Geometry: final body of the model. Coordinates: model frame, mm. A direction names the side the tool comes from. Give positions to 0.01 mm unless a question says otherwise; leave off trailing zeros. Write each loop counter-clockwise with the first axis right and the second up, starting at its lowest first coordinate (ties: lowest second). Pieces come first, ordered by that corner, then holes. Notation, with made-up numbers: (67.25, -11) -> (79.25, -11) arc R12 cw to (79.25, -3) -> close; hole circle Ø11 at (77, -12.5). An arc over 180 degrees is marked (long way). Answer as a JSON object with one key per item and string values.
from build123d import *

# Parameters (mm, degrees)
SKETCH_1_W           = 300
SKETCH_1_H           = 30
EXTRUDE_1_DEPTH      = 20
EXTRUDE_2_DEPTH      = 28
EXTRUDE_2_DEPTH_BACK = 328
SKETCH_3_R           = 4
CUT_EXTRUDE_1_DEPTH  = 182.614977356
SKETCH_3_3_R         = 6
SKETCH_3_3_R_2       = 4
CUT_EXTRUDE_2_DEPTH  = 182.614977356
SKETCH_3_4_R         = 13.5
SKETCH_3_4_R_2       = 13.25
SKETCH_3_4_R_3       = 6
CUT_EXTRUDE_3_DEPTH  = 182.614977356
SKETCH_3_5_R         = 2.4
CUT_EXTRUDE_4_DEPTH  = 4.5
SKETCH_3_6_R         = 2.4
CUT_EXTRUDE_5_DEPTH  = 5


with BuildPart() as part:
    # Sketch 1 → Extrude 1 (new body)
    with BuildSketch(Plane.XY):
        with Locations((0, 15)):
            Rectangle(SKETCH_1_W, SKETCH_1_H)
    extrude(amount=EXTRUDE_1_DEPTH)

    # Sketch 2 → Extrude 2 (add, two sides: drawn at the far end of the back side and taken through both)
    with BuildSketch(Plane.ZY.offset(150).offset(-EXTRUDE_2_DEPTH_BACK)):
        with BuildLine():
            Line((0, 20), (0, 10))
            ThreePointArc((0, 10), (5, 15), (0, 20))
        make_face()
    extrude(amount=EXTRUDE_2_DEPTH + EXTRUDE_2_DEPTH_BACK)

    # Sketch 3 → Cut-Extrude 1 (cut, through all)
    with BuildSketch(Plane(origin=(0, 0, 0), x_dir=(-1, 0, 0), z_dir=(0, 0, -1))):
        with Locations((0, 15)):
            Circle(SKETCH_3_R)
    extrude(amount=-CUT_EXTRUDE_1_DEPTH, mode=Mode.SUBTRACT)

    # Sketch 3_3 → Cut-Extrude 2 (cut, through all)
    with BuildSketch(Plane(origin=(0, 0, 0), x_dir=(-1, 0, 0), z_dir=(0, 0, -1))):
        with Locations((0, 15)):
            Circle(SKETCH_3_3_R)
        with Locations((0, 15)):
            Circle(SKETCH_3_3_R_2, mode=Mode.SUBTRACT)
    extrude(amount=-CUT_EXTRUDE_2_DEPTH, mode=Mode.SUBTRACT)

    # Sketch 3_4 → Cut-Extrude 3 (cut, through all)
    # profile 1 of 2: a face of its own
    with BuildSketch(Plane(origin=(0, 0, 0), x_dir=(-1, 0, 0), z_dir=(0, 0, -1))):
        with Locations((0, 15)):
            Circle(SKETCH_3_4_R)
        with Locations((0, 15)):
            Circle(SKETCH_3_4_R_2, mode=Mode.SUBTRACT)
    # profile 2 of 2: a face of its own
    with BuildSketch(Plane(origin=(0, 0, 0), x_dir=(-1, 0, 0), z_dir=(0, 0, -1))):
        with Locations((0, 15)):
            Circle(SKETCH_3_4_R_2)
        with Locations((0, 15)):
            Circle(SKETCH_3_4_R_3, mode=Mode.SUBTRACT)
    extrude(amount=-CUT_EXTRUDE_3_DEPTH, mode=Mode.SUBTRACT)

    # Sketch 3_5 → Cut-Extrude 4 (cut)
    # profile 1 of 2: a face of its own
    with BuildSketch(Plane(origin=(0, 0, 0), x_dir=(-1, 0, 0), z_dir=(0, 0, -1))):
        with BuildLine():
            ThreePointArc((-6.02027027, 2.916691435), (-13.5, 15), (-6.02027027, 27.083308565))
            Line((-6.02027027, 27.083308565), (-20.841216216, 19.699064442))
            ThreePointArc((-20.841216216, 19.699064442), (-23.75, 15), (-20.841216216, 10.300935558))
            Line((-20.841216216, 10.300935558), (-6.02027027, 2.916691435))
        make_face()
        with Locations((-18.5, 15)):
            Circle(SKETCH_3_5_R, mode=Mode.SUBTRACT)
    # profile 2 of 2: a face of its own
    with BuildSketch(Plane(origin=(0, 0, 0), x_dir=(-1, 0, 0), z_dir=(0, 0, -1))):
        with BuildLine():
            Line((20.841216216, 19.699064442), (6.02027027, 27.083308565))
            ThreePointArc((6.02027027, 27.083308565), (11.478755347, 22.105503197), (13.5, 15))
            ThreePointArc((13.5, 15), (11.478755347, 7.894496803), (6.02027027, 2.916691435))
            Line((6.02027027, 2.916691435), (20.841216216, 10.300935558))
            ThreePointArc((20.841216216, 10.300935558), (23.75, 15), (20.841216216, 19.699064442))
        make_face()
        with Locations((18.5, 15)):
            Circle(SKETCH_3_5_R, mode=Mode.SUBTRACT)
    extrude(amount=-CUT_EXTRUDE_4_DEPTH, mode=Mode.SUBTRACT)

    # Sketch 3_6 → Cut-Extrude 5 (cut)
    with BuildSketch(Plane(origin=(0, 0, 0), x_dir=(-1, 0, 0), z_dir=(0, 0, -1))):
        with Locations((-18.5, 15)):
            Circle(SKETCH_3_6_R)
        with Locations((18.5, 15)):
            Circle(SKETCH_3_6_R)
    extrude(amount=-CUT_EXTRUDE_5_DEPTH, mode=Mode.SUBTRACT)


solid = part.part
Q1. Cut plane A-A (x = 0). Return the cut outline in (y, z).
Values:
{"outline": "(0, 0) -> (1.5, 0) -> (1.5, 20) -> (0, 20) -> close; (28.5, 0) -> (30, 0) -> (30, 20) -> (28.5, 20) -> close"}
Q2. Material intervals for L1, parallel to Y at x = -18.5, z = 4.85; L2, parallel to X at y = 10.75, z = 17; L3, parallel to Z at x = -17.5, y = 15.75, sorted ascending. Write a range as from..to.
Values:
{"L1": "0..12.6, 17.4..30", "L2": "-150..-12.81, 12.81..150", "L3": "5..20"}
Q3. Set-up query: faces 4 (the cylindrical face through (164, 15, 5)), 5 (the cylindrical face through (-164, 15, 5)), 6 (the flat face through (-13.53, 23.34, 2.22)), 7 (the flat face through (2, 29, 0)). Return all of +Z, -Z, +X, -X, +Y, -Y with unobstructed straight access to the full face (end or side cutting, diameter ignored); none if empty.
Values:
{"face 4": "+Z, +X", "face 5": "+Z, -X", "face 6": "-Z", "face 7": "-Z, +X, -X, +Y, -Y"}
Q4. Mould query, pull axis X, two halves, no side actions, for faces 1 (the flat face through (15.6, 15.1, 4.5)), 2 (the flat face through (-2, 29, 20)), 3 (the flat face through (-150, 15, 10)). Classes: pulls with the +X half, pulls with the -X half, needs draft (parallel to the pull), parting line crosses it, or undercut.
Values:
{"face 1": "undercut", "face 2": "needs draft", "face 3": "pulls with the -X half"}
Q5. Cut plane C-C (x = -153.5). Return the cut outline in (y, z).
Values:
{"outline": "(10, 0) -> (20, 0) arc R5 ccw to start"}
Q6. First-contact query: P1, Ø10, axis at y = 22, z = 12, coming from the +X side; P2, Ø10, axis at y = 5, z = 12.5, coming from the -X side; P3, Ø9, axis at x = -15, y = 14.5, coming from the -Z side. Flat tips, straight axial feed; report the tip coordinate or a pass-through.
Values:
{"P1": "x = 150", "P2": "x = -150", "P3": "z = 4.5"}
Q7. Cut plane B-B (z = 12.75). Return the cut outline in (x, y), and give its area (3 significant figures).
Values:
{"outline": "(-150, 0) -> (150, 0) -> (150, 30) -> (-150, 30) -> close; hole circle Ø27 at (0, 15)", "area": "8,430 mm²"}
